Verification items for the finished model (mm, model axes). Face numbers are marked on the shaded views. A direction names the side the tool comes from. Give positions to 0.01 mm unless a question says otherwise; leave off trailing zeros. Loops run counter-clockwise (first coordinate to the right, second up) from the corner with the lowest first, then second, coordinate; pieces in that order, holes last. Notation, with made-up numbers: (49, 69.5) - (67, 69.5) arc R8 cw to (67, 79.5) - close; hole circle Ø7 at (62.25, 15.5). An arc over 180 degrees is marked (long way). Answer in a Markdown table with one row per item.
```python
from build123d import *

# Parameters (mm, degrees)
F1_DEPTH = 15
F2_R     = 6.5
F3_DEPTH = 116.569542
F4_R     = 6.5
F5_DEPTH = 116.569542


with BuildPart() as f1:
    # F0 (on Top) → F1 (new body)
    with BuildSketch(Plane.XY):
        Polygon((-48.284271, 20), (-48.284271, -20), (-20, -48.284271), (20, -48.284271), (48.284271, -20), (48.284271, 20), (20, 48.284271), (-20, 48.284271), align=None)
        Polygon((-18.757359, -45.284271), (-45.284271, -18.757359), (-45.284271, -11.257359), (-45.284271, 18.757359), (-18.757359, 45.284271), (-11.257359, 45.284271), (18.757359, 45.284271), (45.284271, 18.757359), (45.284271, 11.257359), (45.284271, -18.757359), (18.757359, -45.284271), (11.257359, -45.284271), align=None, mode=Mode.SUBTRACT)
        Polygon((-18.106602, 0), (-18.106602, -7.5), (-7.5, -18.106602), (0, -18.106602), (7.5, -18.106602), (18.106602, -7.5), (18.106602, 0), (18.106602, 7.5), (7.5, 18.106602), (0, 18.106602), (-7.5, 18.106602), (-18.106602, 7.5), align=None)
        Polygon((-6.257359, -15.106602), (-15.106602, -6.257359), (-15.106602, 6.257359), (-6.257359, 15.106602), (6.257359, 15.106602), (15.106602, 6.257359), (15.106602, -6.257359), (6.257359, -15.106602), align=None, mode=Mode.SUBTRACT)
        Polygon((-45.284271, -11.257359), (-45.284271, -18.757359), (-18.106602, -7.5), (-18.106602, 0), align=None)
        Polygon((-11.257359, 45.284271), (-18.757359, 45.284271), (-7.5, 18.106602), (0, 18.106602), align=None)
        Polygon((18.106602, 0), (45.284271, 11.257359), (45.284271, 18.757359), (18.106602, 7.5), align=None)
        Polygon((0, -18.106602), (11.257359, -45.284271), (18.757359, -45.284271), (7.5, -18.106602), align=None)
    extrude(amount=F1_DEPTH)

    # F2 (on face) → F3 (cut, through all)
    with BuildSketch(Plane(origin=(34.142136, -34.142136, 0), x_dir=(0.707107, 0.707107, 0), z_dir=(0.707107, -0.707107, 0))):
        with Locations((0, 7.5)):
            Circle(F2_R)
    extrude(amount=-F3_DEPTH, mode=Mode.SUBTRACT)

    # F4 (on face) → F5 (cut, through all)
    with BuildSketch(Plane(origin=(-34.142136, -34.142136, 0), x_dir=(0.707107, -0.707107, 0), z_dir=(-0.707107, -0.707107, 0))):
        with Locations((0, 7.5)):
            Circle(F4_R)
    extrude(amount=-F5_DEPTH, mode=Mode.SUBTRACT)


solid = f1.part
```
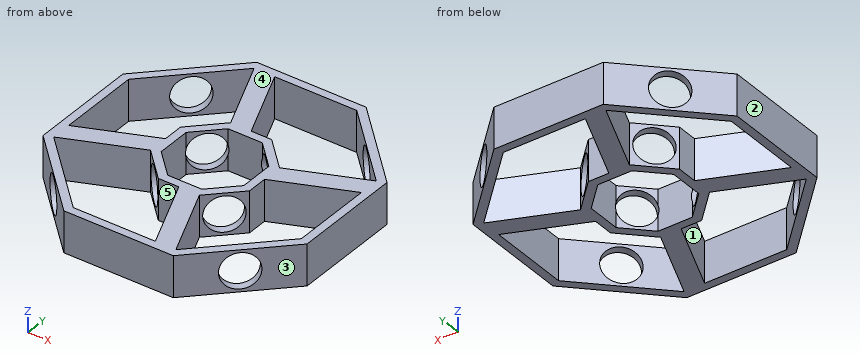
Q1. Thickness scan on line 1 (Y direction, x = 42, z = 5.5); line 2 (Y direction, x = 4.5, z = 13.75); line 3 (X direction, y = 27.5, z = 6.25). Record the ranges inside material, lowest first.
Completed:
| item | result |
|---|---|
| line 1 | -26.28 to -22.04, 9.9 to 17.4, 22.04 to 26.28 |
| line 2 | -48.28 to -45.28, -28.97 to -15.11, 15.11 to 18.11, 45.28 to 48.28 |
| line 3 | -40.78 to -36.54, -11.39 to -3.89, 36.54 to 40.78 |
Q2. Sectioned sample at C-C (z = 4.25). Give the number of separate pieces and of enclosed holes in the cut face, and give its area (3 significant figures).
Completed:
| item | result |
|---|---|
| separate pieces | 4 |
| enclosed holes | 0 |
| area | 1,810 mm^2 |
Q3. Tool access check on the marked faces 4 and 5. Record the directions out of +Z, -Z, +X, -X, +Y, -Y that give a thin tool (end or side, any length) a straight path to the whole face; none if there is none.
Completed:
| item | result |
|---|---|
| face 4 | +Z, +X, -X, +Y, -Y |
| face 5 | +Z, -Z |
Q4. Draft check along X on the marked faces 1, 2 and 3. Enter one of: +X half, -X half, draft (parallel to the pull), parting line (faces both ways), or undercut.
Completed:
| item | result |
|---|---|
| face 1 | undercut |
| face 2 | -X half |
| face 3 | +X half |
Q5. Sectioned sample at B-B (y = -22). Record the cut outline in (x, z), and give its area (3 significant figures).
Completed:
| item | result |
|---|---|
| outline | (-46.28, 0) - (-42.04, 0) - (-42.04, 15) - (-46.28, 15) - close; (1.61, 0) - (9.11, 0) - (9.11, 15) - (1.61, 15) - close; (42.04, 0) - (46.28, 0) - (46.28, 15) - (42.04, 15) - close |
| area | 240 mm^2 |
Q6. Sectioned sample at A-A (y = -4). Record the cut outline in (x, z), and give its area (3 significant figures).
Completed:
| item | result |
|---|---|
| outline | (-48.28, 0) - (-45.28, 0) - (-45.28, 15) - (-48.28, 15) - close; (-27.76, 0) - (-15.11, 0) - (-15.11, 15) - (-27.76, 15) - close; (15.11, 0) - (18.11, 0) - (18.11, 15) - (15.11, 15) - close; (45.28, 0) - (48.28, 0) - (48.28, 15) - (45.28, 15) - close |
| area | 325 mm^2 |
Q7. Go/stop test with flat-tipped pins: P1, Ø8, axis at x = 33.5, y = -28, coming from the -Z side; P2, Ø4, axis at y = -33, z = 2, coming from the -X side; P3, Ø4, axis at y = 36, z = 13, coming from the -X side. Record where each tip stops, or that it passes through.
Completed:
| item | result |
|---|---|
| P1 | z = 0 |
| P2 | x = -37.28 |
| P3 | x = -34.02 |
